The listing builds one solid part. Answer for the finished solid, in the listing's coordinates (mm). Round coordinates to 2 decimals unless told otherwise and drop trailing zeros. Write each loop counter-clockwise with the first axis right and the second up, starting at its lowest first coordinate (ties: lowest second). Pieces come first, ordered by that corner, then holes. Notation, with made-up numbers: (-7.75, 47) - (9.25, 47) arc R30 cw to (9.25, 75) - close; hole circle Ø8 at (-27, 47.5). An arc over 180 degrees is marked (long way). Answer as CSV lines item,"result". Start each with the question number.
Item 1: Straight lines are drawn through the part: line 1 along Y through (x, z) = (-75, 0.2); line 2 along X through (y, z) = (1.5, 3.35); line 3 along Y through (x, z) = (-45, 0.4). For each, find the intervals that lie inside material, in ascending order. Write a range as [from, to].
Item 2: A cutting plane is placed at B-B on z = 3.2. Determine the outline of the cut face in (x, y), and give its area (3 significant figures).
Item 3: A flat-ended cylindrical pin translates along its axis: pin 1 (8 mm diameter, centred on x = 75, y = 30, fed in from +Z). Find the tip coordinate at first contact, or state that the pin passes through.
Item 4: A cutting plane is placed at C-C on y = 0. Determine the outline of the cut face in (x, z), and give its area (3 significant figures).
Item 5: A cutting plane is placed at A-A on x = -75. Determine the outline of the cut face in (y, z), and give its area (3 significant figures).
Item 6: A cutting plane is placed at D-D on x = 45. Determine the outline of the cut face in (y, z), and give its area (3 significant figures).
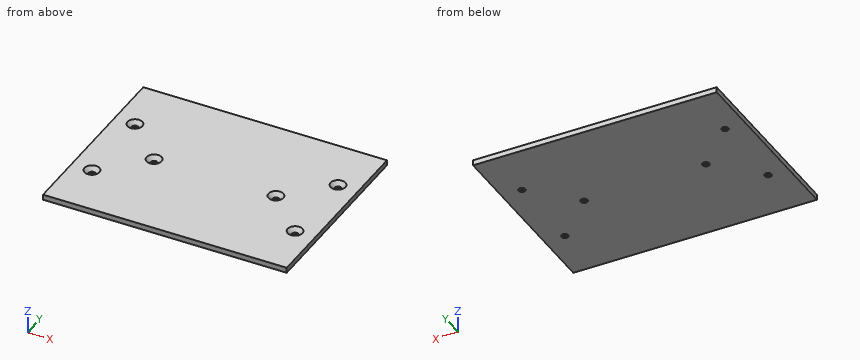
```python
from build123d import *

# Parameters (mm, degrees)
SKETCH1_W           = 180
SKETCH1_H           = 140
BOSS_EXTRUDE1_DEPTH = 4
CUT_EXTRUDE1_REACH  = 116.088
SKETCH2_R           = 2.5
CHAMFER1_SIZE       = 3


with BuildPart() as part:
    # Sketch1 → Boss-Extrude1 (new body)
    with BuildSketch(Plane.XY):
        Rectangle(SKETCH1_W, SKETCH1_H)
    extrude(amount=BOSS_EXTRUDE1_DEPTH)

    # Sketch2 → Cut-Extrude1 (cut, up to next)
    with BuildSketch(Plane(origin=(0, 0, 0), x_dir=(-1, 0, 0), z_dir=(0, 0, -1)), mode=Mode.PRIVATE) as cut_extrude1_sk1:
        with Locations((-75, 30)):
            Circle(SKETCH2_R)
    cut_extrude1_tool1 = extrude(cut_extrude1_sk1.sketch, amount=-CUT_EXTRUDE1_REACH, mode=Mode.PRIVATE) & part.part
    # Sketch2 → Cut-Extrude1 (cut, up to next)
    with BuildSketch(Plane(origin=(0, 0, 0), x_dir=(-1, 0, 0), z_dir=(0, 0, -1)), mode=Mode.PRIVATE) as cut_extrude1_sk2:
        with Locations((-75, -30)):
            Circle(SKETCH2_R)
    cut_extrude1_tool2 = extrude(cut_extrude1_sk2.sketch, amount=-CUT_EXTRUDE1_REACH, mode=Mode.PRIVATE) & part.part
    # Sketch2 → Cut-Extrude1 (cut, up to next)
    with BuildSketch(Plane(origin=(0, 0, 0), x_dir=(-1, 0, 0), z_dir=(0, 0, -1)), mode=Mode.PRIVATE) as cut_extrude1_sk3:
        with Locations((75, -30)):
            Circle(SKETCH2_R)
    cut_extrude1_tool3 = extrude(cut_extrude1_sk3.sketch, amount=-CUT_EXTRUDE1_REACH, mode=Mode.PRIVATE) & part.part
    # Sketch2 → Cut-Extrude1 (cut, up to next)
    with BuildSketch(Plane(origin=(0, 0, 0), x_dir=(-1, 0, 0), z_dir=(0, 0, -1)), mode=Mode.PRIVATE) as cut_extrude1_sk4:
        with Locations((75, 30)):
            Circle(SKETCH2_R)
    cut_extrude1_tool4 = extrude(cut_extrude1_sk4.sketch, amount=-CUT_EXTRUDE1_REACH, mode=Mode.PRIVATE) & part.part
    # Sketch2 → Cut-Extrude1 (cut, up to next)
    with BuildSketch(Plane(origin=(0, 0, 0), x_dir=(-1, 0, 0), z_dir=(0, 0, -1)), mode=Mode.PRIVATE) as cut_extrude1_sk5:
        with Locations((45, 0)):
            Circle(SKETCH2_R)
    cut_extrude1_tool5 = extrude(cut_extrude1_sk5.sketch, amount=-CUT_EXTRUDE1_REACH, mode=Mode.PRIVATE) & part.part
    # Sketch2 → Cut-Extrude1 (cut, up to next)
    with BuildSketch(Plane(origin=(0, 0, 0), x_dir=(-1, 0, 0), z_dir=(0, 0, -1)), mode=Mode.PRIVATE) as cut_extrude1_sk6:
        with Locations((-45, 0)):
            Circle(SKETCH2_R)
    cut_extrude1_tool6 = extrude(cut_extrude1_sk6.sketch, amount=-CUT_EXTRUDE1_REACH, mode=Mode.PRIVATE) & part.part
    add(cut_extrude1_tool1.solids().sort_by_distance((75, 30, 0))[0], mode=Mode.SUBTRACT)
    add(cut_extrude1_tool2.solids().sort_by_distance((75, -30, 0))[0], mode=Mode.SUBTRACT)
    add(cut_extrude1_tool3.solids().sort_by_distance((-75, -30, 0))[0], mode=Mode.SUBTRACT)
    add(cut_extrude1_tool4.solids().sort_by_distance((-75, 30, 0))[0], mode=Mode.SUBTRACT)
    add(cut_extrude1_tool5.solids().sort_by_distance((-45, 0, 0))[0], mode=Mode.SUBTRACT)
    add(cut_extrude1_tool6.solids().sort_by_distance((45, 0, 0))[0], mode=Mode.SUBTRACT)

    # Chamfer1
    chamfer1_edges = [part.edges().sort_by_distance(p)[0] for p in [
        (77.5, 30, 4),
        (77.5, -30, 4),
        (-72.5, -30, 4),
        (-72.5, 30, 4),
        (-42.5, 0, 4),
        (47.5, 0, 4),
    ]]
    chamfer(chamfer1_edges, length=CHAMFER1_SIZE)


solid = part.part
```
Geometry says:
1,line 1,"y = [-70, -32.5], [-27.5, 27.5], [32.5, 70]"
1,line 2,"x = [-90, -49.61], [-40.39, 40.39], [49.61, 90]"
1,line 3,"y = [-70, -2.5], [2.5, 70]"
2,outline,"(-90, -70) - (90, -70) - (90, 70) - (-90, 70) - close; hole circle Ø9.4 at (-75, -30); hole circle Ø9.4 at (-75, 30); hole circle Ø9.4 at (-45, 0); hole circle Ø9.4 at (45, 0); hole circle Ø9.4 at (75, -30); hole circle Ø9.4 at (75, 30)"
2,area,"24,800 mm^2"
3,pin 1,"stops at z = 2.5"
4,outline,"(-90, 0) - (-47.5, 0) - (-47.5, 1) - (-50.5, 4) - (-90, 4) - close; (-42.5, 0) - (42.5, 0) - (42.5, 1) - (39.5, 4) - (-39.5, 4) - (-42.5, 1) - close; (47.5, 0) - (90, 0) - (90, 4) - (50.5, 4) - (47.5, 1) - close"
4,area,"662 mm^2"
5,outline,"(-70, 0) - (-32.5, 0) - (-32.5, 1) - (-35.5, 4) - (-70, 4) - close; (-27.5, 0) - (27.5, 0) - (27.5, 1) - (24.5, 4) - (-24.5, 4) - (-27.5, 1) - close; (32.5, 0) - (70, 0) - (70, 4) - (35.5, 4) - (32.5, 1) - close"
5,area,"502 mm^2"
6,outline,"(-70, 0) - (-2.5, 0) - (-2.5, 1) - (-5.5, 4) - (-70, 4) - close; (2.5, 0) - (70, 0) - (70, 4) - (5.5, 4) - (2.5, 1) - close"
6,area,"531 mm^2"
